Work out the finished part from the listing and answer in its coordinate system (mm). A direction names the side the tool comes from. Coordinates: 2 decimals unless noted, no trailing zeros. Order: outer loops, then holes, each group sorted by start corner. A loop starts at its lowest first (then second) coordinate and runs counter-clockwise, first axis right, second up.
1. Flat-ended cylindrical pins translate along their axes: pin 1 Ø15 at (y, z) = (35, -5.5) entering from -X; pin 2 Ø5 at (x, y) = (21, 21) entering from -Z; pin 3 Ø6 at (x, y) = (15, 12) entering from +Z; pin 4 Ø11.5 at (y, z) = (40, 0) entering from +X. Find the tip coordinate at first contact, or state that the pin passes through.
2. A tool of negligible diameter and unlimited length cuts with its end or side. For faces 4 (the flat face through (22, 25, 15)), 5 (the flat face through (22, 25, -15)), 6 (the cylindrical face through (18.4, 4.39, 20.98)), from which of +Z, -Z, +X, -X, +Y, -Y can it reach the whole face along a straight path? Write none if from no direction.
3. Find the intervals of material crossed by probe 1 along Z at (x, y) = (20.75, 0); probe 2 along Z at (x, y) = (7.75, 0); probe 3 along Y at (x, z) = (6.25, -20), in increasing order.
4. The part is cut by section A-A, the plane z = -20. Give the vertices of the cut face in (x, y).
5. The part is cut by section B-B, the plane x = 23. Give the vertices of the cut face in (y, z) (3 decimals).
6. The part is cut by section D-D, the plane x = 19.5. Give the vertices of the cut face in (y, z) (3 decimals), then the cut area to 3 significant figures.
7. Determine the mould class of faces 1 (the flat face through (11, 2, 18)), 2 (the flat face through (13, 0, -27.5)), 3 (the flat face through (10, -7.5, 0)) for opening direction Y: +Y half, -Y half, draft (parallel to the pull), parting line (faces both ways), or undercut.
8. The part is cut by section C-C, the plane y = 40. Give the vertices of the cut face in (x, z) (3 decimals), then the cut area to 3 significant figures.
Solid Edge part; units mm, degrees
sketch "Sketch1" plane through (0, 0, 0) normal (0, 0, 1) x (1, 0, 0)
  line L0 (0, 7.5) -> (0, -7.5)
  line L1 (0, -7.5) -> (21, -7.5)
  line L2 (21, -7.5) -> (26, -2.5)
  line L3 (26, -2.5) -> (26, 55)
  line L4 (26, 55) -> (18, 55)
  line L5 (18, 55) -> (18, 12.5)
  line L6 (18, 12.5) -> (16, 7.5)
  line L7 (16, 7.5) -> (0, 7.5)
  dimension "D1" = 26
  dimension "D2" = 21
  dimension "D3" = 21
  dimension "D4" = 18
  dimension "D5" = 18
extrude "Protrusion1" add sketch "Sketch1" along normal mid plane 30
hole "Hole_3" at (26, 40, 0) direction (-1, 0, 0) diameter 12.6 end up to next
hole "Hole_4" at (26, 40, 11.25) direction (-1, 0, 0) diameter 3.85 end up to next
hole "Hole1" at (26, 40, -11.25) direction (-1, 0, 0) diameter 3.85 end up to next
chamfer "Chamfer_2" distance 1 angle 60 3 edges at (26, 40, -9.325) (26, 40, 13.175) (26, 40, 6.3) measured on face at (26, 6.5083, 9.7)
hole "Hole_6" at (26, -1.5595, 7.5) direction (-1, 0, 0) diameter 10 end up to next
hole "Hole2" at (26, -1.5595, -7.5) direction (-1, 0, 0) diameter 10 end up to next
sketch "Sketch2" plane through (11.5, 23.75, 0) normal (0, 0, 1) x (1, 0, 0)
  line L0 (-11.5, -31.25) -> (14.5, -31.25)
  line L1 (14.5, -31.25) -> (14.5, -16.25)
  line L2 (14.5, -16.25) -> (-11.5, -16.25)
  line L3 (-11.5, -16.25) -> (-11.5, -31.25)
extrude "Protrusion2" add sketch "Sketch2" along normal mid plane 55
sketch "Sketch3" plane through (11.5, 23.75, 15) normal (0, 0, 1) x (1, 0, 0)
  line L0 (-11.5, -16.25) -> (-10, -16.25)
  line L1 (-10, -16.25) -> (-11.5, -20.25)
  line L2 (-11.5, -20.25) -> (-11.5, -16.25)
  dimension "D1" = 11.5
  dimension "D2" = 11.5
extrude "ExtrudedCutout_3" cut sketch "Sketch3" along normal mid plane 94
sketch "Sketch4" plane through (11.5, 0, 27.5) normal (0, 0, 1) x (1, 0, 0)
  line L0 (14.5, -7.5) -> (14.5, -2.5)
  line L1 (14.5, -2.5) -> (9.5, -7.5)
  line L2 (9.5, -7.5) -> (14.5, -7.5)
  dimension "D1" = 14.5
extrude "Cutout1" cut sketch "Sketch4" against normal through all
hole "Hole_8" at (26, 0, 20) direction (-1, 0, 0) diameter 4.8 end up to next counterbore diameter 9 counterbore depth 15
hole "Hole3" at (26, 0, -20) direction (-1, 0, 0) diameter 4.8 end up to next counterbore diameter 9 counterbore depth 15
fillet "Round1" radius 12 2 edges at (22, 55, 15) (22, 55, -15)
properties material "Polyethylene, low density"
Geometry says:
1. pin 1: stops at x = 18
1. pin 2: stops at z = -15
1. pin 3: stops at z = 15
1. pin 4: passes through
2. face 4: +Z, +X, -X, +Y
2. face 5: -Z, +X, -X, +Y
2. face 6: +X
3. probe 1: z = -27.5 to -24.5, -15.5 to 15.5, 24.5 to 27.5
3. probe 2: z = -27.5 to -22.4, -17.6 to 17.6, 22.4 to 27.5
3. probe 3: y = -7.5 to -2.4, 2.4 to 7.5
4. outline: (0, -7.5) - (21, -7.5) - (24, -4.5) - (11, -4.5) - (11, -2.4) - (0, -2.4) - close; (0, 2.4) - (11, 2.4) - (11, 4.5) - (26, 4.5) - (26, 7.5) - (1.5, 7.5) - (0, 3.5) - close
5. outline: (-5.5, -27.5) - (7.5, -27.5) - (7.5, -15) - (43, -15) arc R12 ccw to (55, -3) - (55, 3) arc R12 ccw to (43, 15) - (7.5, 15) - (7.5, 27.5) - (-5.5, 27.5) - close; hole circle Ø9 at (0, -20); hole circle Ø9 at (0, 20); hole circle Ø12.6 at (40, 0); hole circle Ø3.85 at (40, -11.25); hole circle Ø3.85 at (40, 11.25)
6. outline: (-7.5, -27.5) - (7.5, -27.5) - (7.5, -15) - (43, -15) arc R12 ccw to (55, -3) - (55, 3) arc R12 ccw to (43, 15) - (7.5, 15) - (7.5, 27.5) - (-7.5, 27.5) - close; hole circle Ø9 at (0, -20); hole circle Ø9 at (0, 20); hole circle Ø12.6 at (40, 0); hole circle Ø3.85 at (40, -11.25); hole circle Ø3.85 at (40, 11.25)
6. area: 1,910 mm2
7. face 1: undercut
7. face 2: draft
7. face 3: -Y half
8. outline: (18, -15) - (26, -15) - (26, -14.175) - (24.268, -13.175) - (18, -13.175) - close; (18, -9.325) - (24.268, -9.325) - (26, -8.325) - (26, -7.3) - (24.268, -6.3) - (18, -6.3) - close; (18, 6.3) - (24.268, 6.3) - (26, 7.3) - (26, 8.325) - (24.268, 9.325) - (18, 9.325) - close; (18, 13.175) - (24.268, 13.175) - (26, 14.175) - (26, 15) - (18, 15) - close
8. area: 72.4 mm2
